Can you work these out from the model? Positions are in its coordinate system, mm. A direction names the side the tool comes from. Round coordinates to 2 decimals unless told otherwise and drop trailing zeros. Write each loop counter-clockwise with the first axis right and the second up, starting at its lowest first coordinate (ties: lowest second). Pieces come first, ordered by that corner, then holes. Notation, with made-up numbers: M 58.25,-22 L 115.25,-22 A11 cw 115.25,-6 Z; hole C -28,52 d4. An arc over 180 degrees is marked long. Answer as a JSON object with one key per item and string values. Group by question number.
1) Suppose I cut it at A-A, the plane y = -12. Write out the boundary of the cut face in (x, z), and give its area (3 significant figures).
2) Suppose I cut it at C-C, the plane x = 50. Write out the boundary of the cut face in (y, z), and give its area (3 significant figures).
3) Suppose I cut it at B-B, the plane z = 22. Write out the boundary of the cut face in (x, y).
4) Suppose I cut it at D-D, the plane y = -4. Write out the boundary of the cut face in (x, z), and give its area (3 significant figures).
5) I'm going to push flat-ended pins straight in: pin 1 Ø1.5 at (x, y) = (57, -13) entering from +Z; pin 2 Ø9 at (x, y) = (10, -36) entering from +Z; pin 3 Ø7.5 at (x, y) = (34, -15.5) entering from -Z; pin 4 Ø1 at (y, z) = (-36.5, 22) entering from -X. Where does each tip first touch, or does it pass through?
6) If we mould it in two halves opening along Y, with no side actions, what happens to faces 4 (the flat face through (35, -41, 20)), 5 (the flat face through (45, -20, 8)), 6 (the cylindrical face through (43.367, -4.056, 28.083))? For each: +Y half, -Y half, draft (parallel to the pull), parting line (faces both ways), or undercut.
7) On a 3-axis mill with a long thin cutter (end or side, diameter ignored), from which of +Z, -Z, +X, -X, +Y, -Y can I reach the whole of each face in a straight line? I mean faces 1 (the flat face through (11, -37, 16)), 2 (the flat face through (38, -20, 43)), 3 (the flat face through (89.712, -20.787, 5.064)). Say none if no direction works.
8) Please list where these lines run through material, in increasing order: L1, parallel to Y at x = 75.5, z = 19; L2, parallel to Z at x = 39, y = -18.5; L3, parallel to Z at x = 76.5, y = -28.5. Write a range as [from, to].
from build123d import *

# Parameters (mm, degrees)
F0_W          = 92
F0_H          = 51
F1_DEPTH      = 41
F2_W          = 22
F2_H          = 35
F3_DEPTH      = 41.001
F5_DEPTH      = 41.001
F6_R          = 9
F7_DEPTH      = 41.001
F8_W          = 25
F8_H          = 35
F9_DEPTH      = 70.001
F9_DEPTH_BACK = 25.4


with BuildPart() as f1:
    # F0 (on Front) → F1 (new body)
    with BuildSketch(Plane.XZ):
        with Locations((46, 25.5)):
            Rectangle(F0_W, F0_H)
    extrude(amount=F1_DEPTH)

    # F2 (on face) → F3 (cut, through all)
    with BuildSketch(Plane.XZ.offset(41)):
        with Locations((11, 33.5)):
            Rectangle(F2_W, F2_H)
    extrude(amount=-F3_DEPTH, mode=Mode.SUBTRACT)

    # F4 (on face) → F5 (cut, through all)
    with BuildSketch(Plane.XZ.offset(41)):
        Polygon((92, 51), (41, 51), (78.8247816226, 29.1618521481), (92, 0), align=None)
    extrude(amount=-F5_DEPTH, mode=Mode.SUBTRACT)

    # F6 (on face) → F7 (cut, through all)
    with BuildSketch(Plane.XZ.offset(41)):
        with Locations((50, 22)):
            Circle(F6_R)
    extrude(amount=-F7_DEPTH, mode=Mode.SUBTRACT)

    # F8 (on face) → F9 (cut, two sides)
    with BuildSketch(Plane(origin=(22, 0, 0), x_dir=(0, -1, 0), z_dir=(-1, 0, 0))) as f9_sk:
        with Locations((20.5, 25.5)):
            Rectangle(F8_W, F8_H)
    extrude(amount=-F9_DEPTH, mode=Mode.SUBTRACT)
    extrude(f9_sk.sketch, amount=F9_DEPTH_BACK, mode=Mode.SUBTRACT)


solid = f1.part
Results:
{
 "1": {"outline": "M 0,0 L 92,0 L 88.39,8 L 0,8 Z; M 22,43 L 54.86,43 L 41,51 L 22,51 Z", "area": "929 mm^2"},
 "2": {"outline": "M -41,0 L 0,0 L 0,13 L -8,13 L -8,8 L -33,8 L -33,13 L -41,13 Z; M -41,31 L -33,31 L -33,43 L -8,43 L -8,31 L 0,31 L 0,45.8 L -41,45.8 Z", "area": "715 mm^2"},
 "3": {"outline": "M 22,-41 L 41,-41 L 41,-33 L 22,-33 Z; M 22,-8 L 41,-8 L 41,0 L 22,0 Z; M 59,-41 L 82.06,-41 L 82.06,-33 L 59,-33 Z; M 59,-8 L 82.06,-8 L 82.06,0 L 59,0 Z"},
 "4": {"outline": "M 0,0 L 92,0 L 78.82,29.16 L 41,51 L 22,51 L 22,16 L 0,16 Z; hole C 50,22 d18", "area": "2,770 mm^2"},
 "5": {"pin 1": "z = 8", "pin 2": "z = 16", "pin 3": "z = 0", "pin 4": "x = 22"},
 "6": {"face 4": "-Y half", "face 5": "undercut", "face 6": "draft"},
 "7": {"face 1": "+Z, -X, +Y, -Y", "face 2": "+X, -X", "face 3": "+Z, +X, +Y, -Y"},
 "8": {"L1": "[-41, -33], [-8, 0]", "L2": "[0, 8], [43, 51]", "L3": "[0, 8]"}
}
